Part print with two shaded views. Sizes in mm from the minimum x, y, z corner. A direction names the side the tool comes from. Round coordinates to 2 decimals unless told otherwise and drop trailing zeros. Order: outer loops, then holes, each group sorted by start corner. A loop starts at its lowest first (then second) coordinate and runs counter-clockwise, first axis right, second up. Notation, with made-up numbers: (-26, -29.75) -> (33, -29.75) arc R20 ccw to (33, -5.75) -> close; hole circle Ø4 at (-32.75, 10). An arc over 180 degrees is marked (long way). Answer as a JSON object with one key per item and string values.
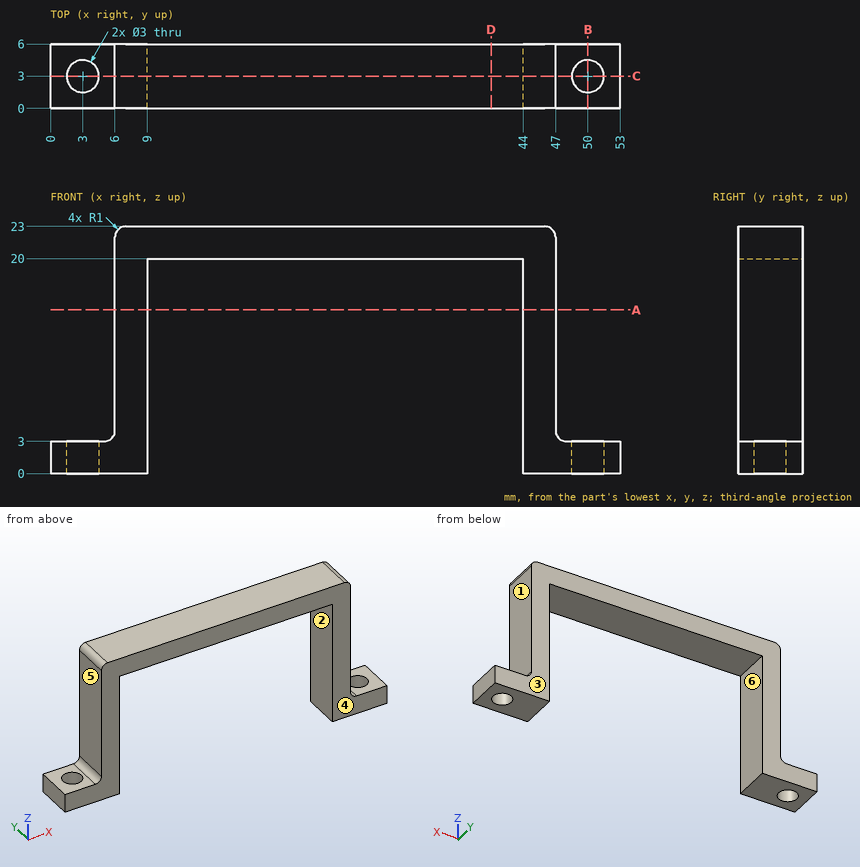
1) Cut at C-C, the plane y = 3. Give the cut face in (x, z), plus the area to 3 significant figures.
Checked values:
{"outline": "(0, 0) -> (1.5, 0) -> (1.5, 3) -> (0, 3) -> close; (4.5, 0) -> (9, 0) -> (9, 20) -> (44, 20) -> (44, 0) -> (48.5, 0) -> (48.5, 3) -> (48, 3) arc R1 cw to (47, 4) -> (47, 22) arc R1 ccw to (46, 23) -> (7, 23) arc R1 ccw to (6, 22) -> (6, 4) arc R1 cw to (5, 3) -> (4.5, 3) -> close; (51.5, 0) -> (53, 0) -> (53, 3) -> (51.5, 3) -> close", "area": "261 mm²"}
2) Probe L1, parallel to X at y = 2.45, z = 12; L2, parallel to X at y = 2.7, z = 1.75; L3, parallel to X at y = 5.6, z = 1.5. List the from-to ranges inside material, lowest first. Write a range as from..to.
Checked values:
{"L1": "x = 6..9, 44..47", "L2": "x = 0..1.53, 4.47..9, 44..48.53, 51.47..53", "L3": "x = 0..9, 44..53"}
3) Pull direction X, two halves, no side cores. Call the marked faces 1, 2 and 3: pulls with the +X half, pulls with the -X half, needs draft (parallel to the pull), parting line crosses it, or undercut.
Checked values:
{"face 1": "pulls with the +X half", "face 2": "undercut", "face 3": "needs draft"}
4) Which spindle directions (+Z, -Z, +X, -X, +Y, -Y) get a long thin tool onto all of the face, cutting with end or side? Do the marked faces 4, 5 and 6. Say none if no direction does.
Checked values:
{"face 4": "+Z, -Z, +X, -X, -Y", "face 5": "+Z, -X, +Y, -Y", "face 6": "-Z, +Y, -Y"}
5) Cut at A-A, the plane z = 15.25. Give the cut face in (x, y), plus the area to 3 significant figures.
Checked values:
{"outline": "(6, 0) -> (9, 0) -> (9, 6) -> (6, 6) -> close; (44, 0) -> (47, 0) -> (47, 6) -> (44, 6) -> close", "area": "36.0 mm²"}
6) Cut at D-D, the plane x = 41. Give the cut face in (y, z).
Checked values:
{"outline": "(0, 20) -> (6, 20) -> (6, 23) -> (0, 23) -> close"}
7) Cut at B-B, the plane x = 50. Give the cut face in (y, z), plus the area to 3 significant figures.
Checked values:
{"outline": "(0, 0) -> (1.5, 0) -> (1.5, 3) -> (0, 3) -> close; (4.5, 0) -> (6, 0) -> (6, 3) -> (4.5, 3) -> close", "area": "9.00 mm²"}
8) Flat gauge pins, fed straight in: pin 1 Ø2.5 at (x, y) = (50, 3) entering from +Z; pin 2 Ø1.5 at (x, y) = (51, 4) entering from +Z. Where does each tip first touch, or does it go through?
Checked values:
{"pin 1": "passes through", "pin 2": "stops at z = 3"}
